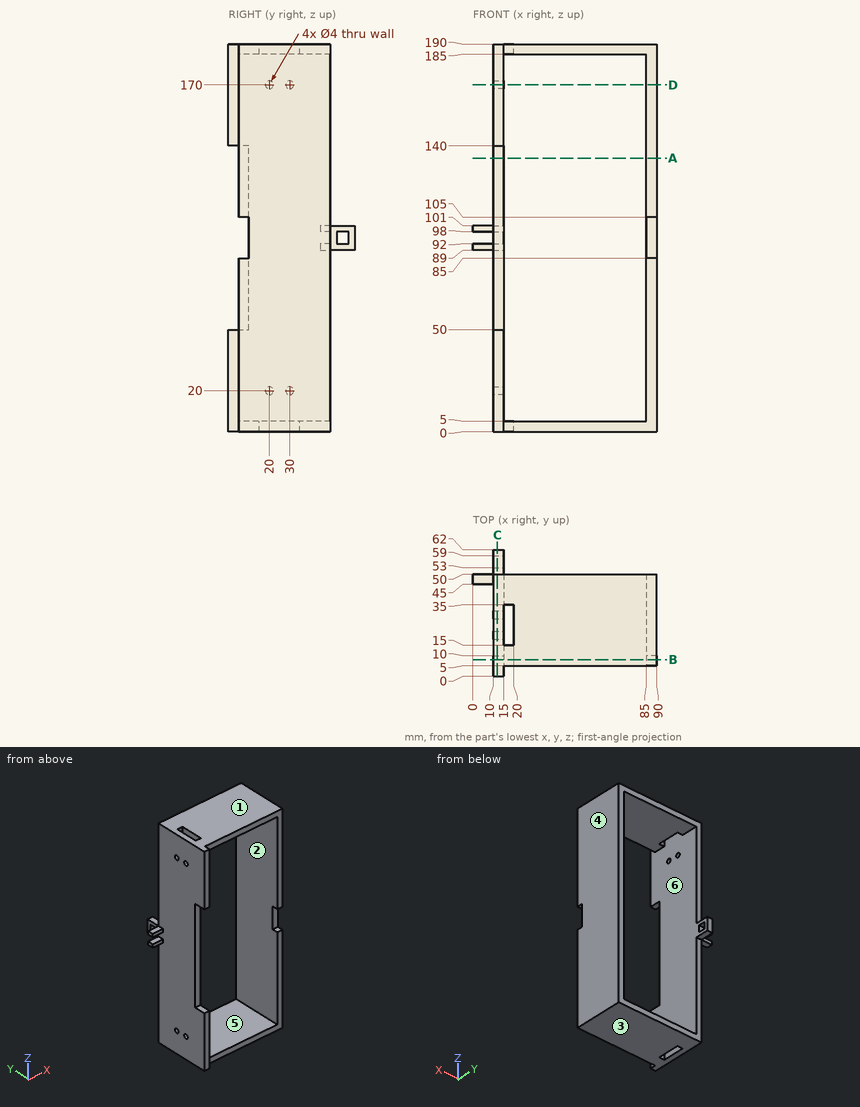
Print and shaded views of the part. All mm, measured from the part's lowest x, y and z. A direction names the side the tool comes from. Give positions to 0.01 mm unless a question says otherwise; leave off trailing zeros. Order: outer loops, then holes, each group sorted by start corner. A loop starts at its lowest first (then second) coordinate and runs counter-clockwise, first axis right, second up. Notation, with made-up numbers: (13.25, 14.5) - (18.25, 14.5) arc R21 ccw to (18.25, 22.5) - close; hole circle Ø1 at (-12, -32.75). An arc over 180 degrees is marked (long way). Use a Markdown table: item, result.
1) 3-axis set-ups, long thin cutter, end or side, ignore diameter. For the marked faces 1 and 2: which of +Z, -Z, +X, -X, +Y, -Y reach the whole face in a straight line?
Checked values:
| item | result |
|---|---|
| face 1 | +Z, +X, -X, +Y, -Y |
| face 2 | +Y, -Y |
2) Probe L1, parallel to Y at x = 12.5, z = 20; L2, parallel to X at y = 24, z = 156.5; L3, parallel to Z at x = 78.5, y = 39. List the from-to ranges inside material, lowest first. Write a range as from..to.
Checked values:
| item | result |
|---|---|
| L1 | 0..18, 22..28, 32..50 |
| L2 | 10..15, 85..90 |
| L3 | 0..5, 185..190 |
3) Saw through at D-D on z = 170. List the corners of the cut face in (x, y).
Checked values:
| item | result |
|---|---|
| outline | (10, 0) - (15, 0) - (15, 18) - (10, 18) - close; (10, 22) - (15, 22) - (15, 28) - (10, 28) - close; (10, 32) - (15, 32) - (15, 50) - (10, 50) - close; (85, 5) - (90, 5) - (90, 50) - (85, 50) - close |
4) Saw through at B-B on y = 8. List the corners of the cut face in (x, z), plus the area to 3 significant figures.
Checked values:
| item | result |
|---|---|
| outline | (10, 0) - (90, 0) - (90, 85) - (85, 85) - (85, 5) - (15, 5) - (15, 50) - (10, 50) - close; (10, 140) - (15, 140) - (15, 185) - (85, 185) - (85, 105) - (90, 105) - (90, 190) - (10, 190) - close |
| area | 2,050 mm² |
5) Saw through at C-C on x = 12. List the corners of the cut face in (y, z).
Checked values:
| item | result |
|---|---|
| outline | (0, 0) - (50, 0) - (50, 89) - (62, 89) - (62, 101) - (50, 101) - (50, 190) - (0, 190) - (0, 140) - (10, 140) - (10, 50) - (0, 50) - close; hole circle Ø4 at (20, 20); hole circle Ø4 at (20, 170); hole circle Ø4 at (30, 20); hole circle Ø4 at (30, 170); hole (53, 92) - (59, 92) - (59, 98) - (53, 98) - close |
6) Two-plate mould, pull along Z, no slides. Class the marked faces 3, 4, 5 and 6: +Z half, -Z half, draft (parallel to the pull), parting line (faces both ways), or undercut.
Checked values:
| item | result |
|---|---|
| face 3 | -Z half |
| face 4 | draft |
| face 5 | undercut |
| face 6 | undercut |
7) Saw through at A-A on z = 134. List the corners of the cut face in (x, y), plus the area to 3 significant figures.
Checked values:
| item | result |
|---|---|
| outline | (10, 10) - (15, 10) - (15, 50) - (10, 50) - close; (85, 5) - (90, 5) - (90, 50) - (85, 50) - close |
| area | 425 mm² |
8) Flat gauge pins, fed straight in: P1, Ø2, axis at y = 20.5, z = 74, coming from the -X side; P2, Ø4, axis at x = 13.5, z = 108.5, coming from the -Y side; P3, Ø2.5, axis at x = 6, z = 90, coming from the +Y side. Where does each tip first touch, or does it go through?
Checked values:
| item | result |
|---|---|
| P1 | x = 10 |
| P2 | y = 10 |
| P3 | y = 50 |
